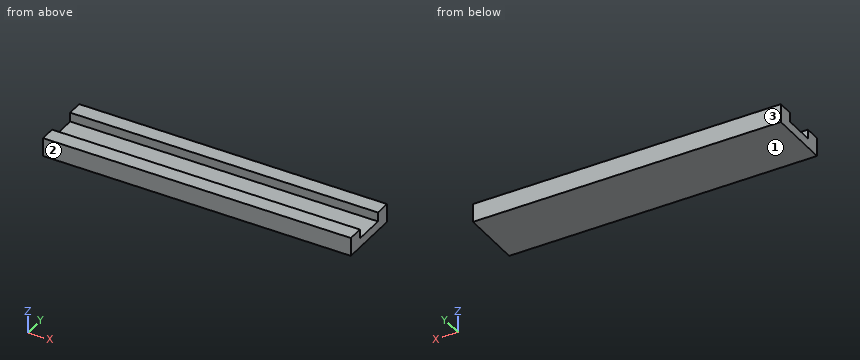
from build123d import *

# Parameters (mm, degrees)
SKETCH_W     = 100
SKETCH_H     = 20
PAD_DEPTH    = 3
SKETCH001_W  = 100
SKETCH001_H  = 5
PAD001_DEPTH = 3


with BuildPart() as part:
    # Sketch → Pad (new body)
    with BuildSketch(Plane.XY):
        Rectangle(SKETCH_W, SKETCH_H)
    extrude(amount=PAD_DEPTH)

    # Sketch001 (on Face6 of Pad) → Pad001 (join)
    with BuildSketch(Plane.XY.offset(3)):
        with Locations((0, 7.5)):
            Rectangle(SKETCH001_W, SKETCH001_H)
        with Locations((0, -7.5)):
            Rectangle(SKETCH001_W, SKETCH001_H)
    extrude(amount=PAD001_DEPTH)


solid = part.part
Source: CAD feature listing. Evaluate the final solid. Frame: model axes, mm. Face numbers are marked on the shaded views. Coordinates: 2 decimals unless noted, no trailing zeros. Loops run counter-clockwise (first coordinate to the right, second up) from the corner with the lowest first, then second, coordinate; pieces in that order, holes last. Notation, with made-up numbers: (89, 67.5) -> (136, 67.5) arc R25 cw to (136, 89.5) -> close; hole circle Ø3 at (87.25, -39). An arc over 180 degrees is marked (long way). Answer in a Markdown table with one row per item. Add a question column.
Q1. Section A-A on z = 5.15. Return the cut outline in (x, y).
Q2. Ray query, line 1 along Y through (x, z) = (41, 4); line 2 along Z through (x, y) = (-45, 2). Return the intervals inside material, ascending.
Q3. Section B-B on x = 7. Return the cut outline in (y, z), and give its area (3 significant figures).
Q4. Section C-C on y = 2.5. Return the cut outline in (x, z), and give its area (3 significant figures).
Q5. Contact query for a flat-ended pin moving along its axis: pin 1 Ø6 at (x, y) = (21, -4.5) entering from +Z. Output: stop coordinate, or through.
Q6. Pull-direction query (Y, two-part tool) for the marked faces 1, 2 and 3; classes: pulls with the +Y half, pulls with the -Y half, needs draft (parallel to the pull), parting line crosses it, or undercut.
Computed values:
| question | item | result |
|---|---|---|
| 1 | outline | (-50, -10) -> (50, -10) -> (50, -5) -> (-50, -5) -> close; (-50, 5) -> (50, 5) -> (50, 10) -> (-50, 10) -> close |
| 2 | line 1 | y = -10 to -5, 5 to 10 |
| 2 | line 2 | z = 0 to 3 |
| 3 | outline | (-10, 0) -> (10, 0) -> (10, 6) -> (5, 6) -> (5, 3) -> (-5, 3) -> (-5, 6) -> (-10, 6) -> close |
| 3 | area | 90.0 mm^2 |
| 4 | outline | (-50, 0) -> (50, 0) -> (50, 3) -> (-50, 3) -> close |
| 4 | area | 300 mm^2 |
| 5 | pin 1 | stops at z = 6 |
| 6 | face 1 | needs draft |
| 6 | face 2 | pulls with the -Y half |
| 6 | face 3 | pulls with the +Y half |
